Check sheet for the modelled part. Datum: model origin and axes. Units: mm. Round coordinates to 2 decimals unless told otherwise and drop trailing zeros. Write each loop counter-clockwise with the first axis right and the second up, starting at its lowest first coordinate (ties: lowest second). Pieces come first, ordered by that corner, then holes.
Item 1: Section check A-A, the plane z = 0.9. Record the cut outline in (x, y), plus the area to 3 significant figures.
Item 2: Section check C-C, the plane y = 17.5. Record the cut outline in (x, z), plus the area to 3 significant figures.
Item 3: Section check B-B, the plane x = 45.5. Record the cut outline in (y, z).
Item 4: Material ranges on line 1 along Y through (x, z) = (0, 1.4); line 2 along Y through (x, z) = (19, 1.2); line 3 along Y through (x, z) = (-33, 0.55), recorded low to high.
Item 5: Depth check by flat-ended pin: pin 1 (2.5 mm diameter, centred on x = 0, y = -42.5, fed in from +Z); pin 2 (1.5 mm diameter, centred on x = -5, z = 1.5, fed in from +Y). Enter the tip coordinate at first touch or a pass-through.
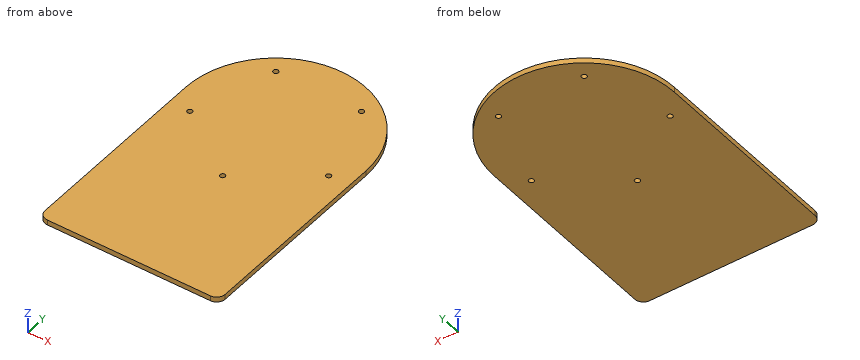
from build123d import *

# Parameters (mm, degrees)
SALIENTE_EXTRUIR1_DEPTH = 3
REDONDEO1_R             = 5
CROQUIS2_R              = 1.5
CORTAR_EXTRUIR1_DEPTH   = 3


with BuildPart() as part:
    # Croquis1 → Saliente-Extruir1 (new body)
    with BuildSketch(Plane.XY):
        with BuildLine():
            ThreePointArc((52.5, 0), (0, -52.5), (-52.5, 0))
            Line((-52.5, 0), (-52.5, -117.5))
            Line((-52.5, -117.5), (52.5, -117.5))
            Line((52.5, -117.5), (52.5, 0))
        make_face()
        with BuildLine():
            ThreePointArc((52.5, 0), (0, 52.5), (-52.5, 0))
            Line((-52.5, 0), (52.5, 0))
        make_face()
        with BuildLine():
            Line((52.5, 0), (-52.5, 0))
            ThreePointArc((-52.5, 0), (0, -52.5), (52.5, 0))
        make_face()
    extrude(amount=SALIENTE_EXTRUIR1_DEPTH)

    # Redondeo1
    redondeo1_edges = [part.edges().sort_by_distance(p)[0] for p in [
        (52.5, -117.5, 1.5),
        (-52.5, -117.5, 1.5),
    ]]
    fillet(redondeo1_edges, radius=REDONDEO1_R)

    # Croquis2 → Cortar-Extruir1 (cut)
    with BuildSketch(Plane.XY.offset(3)):
        with Locations((0, -42.5)):
            Circle(CROQUIS2_R)
        with Locations((-40.419901943, -13.133222261)):
            Circle(CROQUIS2_R)
        with Locations((-24.980873222, 34.383222261)):
            Circle(CROQUIS2_R)
        with Locations((24.980873222, 34.383222261)):
            Circle(CROQUIS2_R)
        with Locations((40.419901943, -13.133222261)):
            Circle(CROQUIS2_R)
    extrude(amount=-CORTAR_EXTRUIR1_DEPTH, mode=Mode.SUBTRACT)


solid = part.part
Values found:
1. outline: (-52.5, -112.5) arc R5 ccw to (-47.5, -117.5) - (47.5, -117.5) arc R5 ccw to (52.5, -112.5) - (52.5, 0) arc R52.5 ccw to (-52.5, 0) - close; hole circle Ø3 at (-40.42, -13.13); hole circle Ø3 at (-24.98, 34.38); hole circle Ø3 at (0, -42.5); hole circle Ø3 at (24.98, 34.38); hole circle Ø3 at (40.42, -13.13)
1. area: 16,600 mm2
2. outline: (-49.5, 0) - (49.5, 0) - (49.5, 3) - (-49.5, 3) - close
2. area: 297 mm2
3. outline: (-117.5, 0) - (26.19, 0) - (26.19, 3) - (-117.5, 3) - close
4. line 1: y = -117.5 to -44, -41 to 52.5
4. line 2: y = -117.5 to 48.94
4. line 3: y = -117.5 to 40.83
5. pin 1: passes through
5. pin 2: stops at y = 52.33
